Design review of the part built by this model. Coordinates are the model's own, in mm. Face numbers are marked on the shaded views. A direction names the side the tool comes from. Coordinates: 2 decimals unless noted, no trailing zeros. Order: outer loops, then holes, each group sorted by start corner. A loop starts at its lowest first (then second) coordinate and runs counter-clockwise, first axis right, second up. Notation, with made-up numbers: (64, 70.25) - (104, 70.25) arc R20 ccw to (104, 94.25) - close; hole circle Ø11 at (58.25, 65). An arc over 180 degrees is marked (long way). Write item = value, one per line. Start each with the question number.
```python
from build123d import *

# Parameters (mm, degrees)
SKETCH_1_W             = 14.3
SKETCH_1_H             = 17
EXTRUDE_1_DEPTH        = 6
SKETCH_3_W             = 0.2
SKETCH_3_H             = 0.2
EXTRUDE_3_DEPTH        = 1.2
PATTERN_LINEAR_1_COUNT = 19
PATTERN_LINEAR_1_PITCH = 0.5
SKETCH_4_W             = 0.3
SKETCH_4_H             = 0.5
EXTRUDE_4_DEPTH        = 6
CUT_EXTRUDE_1_DEPTH    = 10
SKETCH_8_W             = 0.883352336
SKETCH_8_H             = 11.931096145
EXTRUDE_6_DEPTH        = 5.2
CUT_EXTRUDE_4_DEPTH    = 24.382472068
EXTRUDE_7_DEPTH        = 2.1
EXTRUDE_7_DEPTH_BACK   = 5.2
SKETCH_12_W            = 1.5
SKETCH_12_H            = 0.486445161
SKETCH_12_W_2          = 1
SKETCH_13_R            = 0.6
EXTRUDE_8_DEPTH        = 2
SKETCH_15_R            = 1.25
EXTRUDE_9_DEPTH        = 0.4
SKETCH_16_W            = 4.2
SKETCH_16_H            = 9
EXTRUDE_10_DEPTH       = 3.3
FILLET_1_R             = 0.3


with BuildPart() as part:
    # 草图1 → 凸台-拉伸1 (new body)
    with BuildSketch(Plane.XY):
        with Locations((7.15, -8.5)):
            Rectangle(SKETCH_1_W, SKETCH_1_H)
    extrude(amount=EXTRUDE_1_DEPTH)

    # 草图3 → 凸台-拉伸3 (add)
    with BuildSketch(Plane(origin=(14.3, 0, 0), x_dir=(0, 0, -1), z_dir=(1, 0, 0))):
        with Locations((-0.1, -13.9)):
            Rectangle(SKETCH_3_W, SKETCH_3_H)
    extrude_3 = extrude(amount=EXTRUDE_3_DEPTH)

    # 阵列(线性)1: 凸台-拉伸3 ×19
    with Locations(*[(0, i * PATTERN_LINEAR_1_PITCH, 0) for i in range(1, PATTERN_LINEAR_1_COUNT)]):
        add(extrude_3)

    # 草图4 → 凸台-拉伸4 (add)
    with BuildSketch(Plane.XY.offset(6)):
        with Locations((0.15, 0.25)):
            Rectangle(SKETCH_4_W, SKETCH_4_H)
        with Locations((0.15, -17.25)):
            Rectangle(SKETCH_4_W, SKETCH_4_H)
    extrude(amount=-EXTRUDE_4_DEPTH)

    # 草图6 → 切除-拉伸1 (cut)
    with BuildSketch(Plane.ZY):
        Polygon((0.814275945, -1.576993803), (1.814275945, -0.576993803), (5.086945076, -0.576993803), (5.086945076, -16.573920601), (0.814275945, -16.573920601), align=None)
    extrude(amount=-CUT_EXTRUDE_1_DEPTH, mode=Mode.SUBTRACT)

    # 草图8 → 凸台-拉伸6 (add)
    with BuildSketch(Plane.ZY.offset(-10)):
        with Locations((2.941004683, -8.691870864)):
            Rectangle(SKETCH_8_W, SKETCH_8_H)
    extrude(amount=EXTRUDE_6_DEPTH)

    # 草图11 → 切除-拉伸4 (cut, through all)
    with BuildSketch(Plane(origin=(14.3, 0, 0), x_dir=(0, 0, -1), z_dir=(1, 0, 0))):
        Polygon((-2.744957318, 0.690687189), (0.440532754, -2.430132002), (0.440532754, 0.690687189), align=None)
    extrude(amount=-CUT_EXTRUDE_4_DEPTH, mode=Mode.SUBTRACT)

    # 草图12 → 凸台-拉伸7 (add, two sides: drawn at the far end of the back side and taken through both)
    with BuildSketch(Plane(origin=(0, 0, 0), x_dir=(-1, 0, 0), z_dir=(0, 0, -1)).offset(-EXTRUDE_7_DEPTH_BACK)):
        with Locations((-12.05, -16.75677742)):
            Rectangle(SKETCH_12_W, SKETCH_12_H)
        with Locations((-4.8, -16.75677742)):
            Rectangle(SKETCH_12_W_2, SKETCH_12_H)
        with Locations((-4.8, -0.243222581)):
            Rectangle(SKETCH_12_W_2, SKETCH_12_H)
        with Locations((-12.05, -0.243222581)):
            Rectangle(SKETCH_12_W, SKETCH_12_H)
    extrude(amount=EXTRUDE_7_DEPTH + EXTRUDE_7_DEPTH_BACK)

    # 草图13 → 凸台-拉伸8 (add)
    with BuildSketch(Plane(origin=(0, 0, 0), x_dir=(-1, 0, 0), z_dir=(0, 0, -1))):
        with Locations(Location((-4.5, -8.757432115, 0), (0, 0, 180))):
            Circle(SKETCH_13_R)
    extrude(amount=EXTRUDE_8_DEPTH)

    # 草图15 → 凸台-拉伸9 (add)
    with BuildSketch(Plane.ZY):
        with BuildLine():
            Line((6, -2.5), (13.5, -2.5))
            ThreePointArc((13.5, -2.5), (14.914213562, -3.085786438), (15.5, -4.5))
            Line((15.5, -4.5), (15.5, -12.5))
            ThreePointArc((15.5, -12.5), (14.914213562, -13.914213562), (13.5, -14.5))
            Line((13.5, -14.5), (6, -14.5))
            Line((6, -14.5), (6, -2.5))
        make_face()
        with Locations(Location((12.5, -8.5, 0), (0, 0, 270))):
            Circle(SKETCH_15_R, mode=Mode.SUBTRACT)
    extrude(amount=-EXTRUDE_9_DEPTH)

    # 草图16 → 凸台-拉伸10 (add)
    with BuildSketch(Plane.ZY):
        with Locations((3, -8.5)):
            Rectangle(SKETCH_16_W, SKETCH_16_H)
    extrude(amount=EXTRUDE_10_DEPTH)

    # 圆角1
    fillet_1_edges = [part.edges().sort_by_distance(p)[0] for p in [
        (0.3, 0.25, 6),
        (0.3, -17.25, 0),
        (0.3, -17.25, 6),
        (0.3, 0, 4.019978715),
        (0.4, -8.5, 6),
        (0.3, -17, 3),
        (2.3, -17, 0),
        (8.3, -17, 0),
        (13.55, -17, 0),
        (14.3, -17, 3),
        (7.3, -17, 6),
        (14.3, 0, 4.019978715),
        (14.3, -8.5, 6),
        (7.3, 0, 6),
    ]]
    fillet(fillet_1_edges, radius=FILLET_1_R - 0.0001)  # a hair under: the kernel refuses the full size


solid = part.part
```
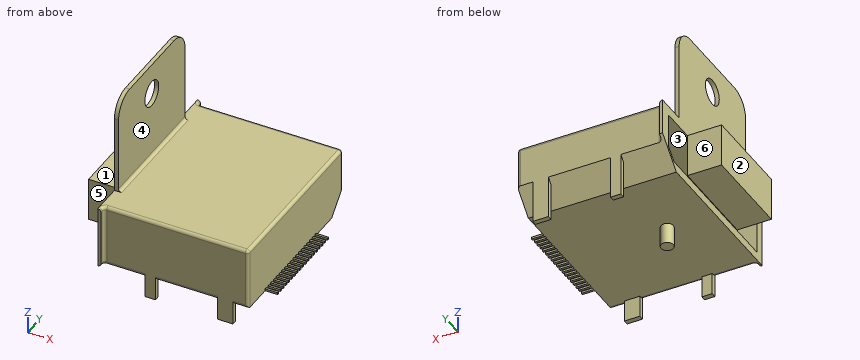
Item 1: For line 1 (Z direction, x = 0.2, y = -8.5); line 2 (Z direction, x = 1.25, y = -9); line 3 (Z direction, x = 8.5, y = -4.5), list the stretches that pass through material, from the lowest coordinate up.
Item 2: For P1, Ø3, axis at y = -13, z = 8, coming from the +X side; P2, Ø0.5, axis at y = -17, z = -1, coming from the +X side; P3, Ø4, axis at x = 13, z = 3.5, coming from the -Y side, all flat-tipped, find the tip position at first contact; note any pin that passes through.
Item 3: Add section D-D on z = -1. Give the boundary of the cut face in (x, y), plus the area to 3 significant figures.
Item 4: Add section C-C on z = 12.5. Give the boundary of the cut face in (x, y).
Item 5: For the marked faces 4, 5 and 6, list the 3-axis set-ups (+Z, -Z, +X, -X, +Y, -Y) from which the entire face can be reached by the end or side of a thin tool; tool diameter is ignored.
Item 6: Add section B-B on x = 2.5. Give the boundary of the cut face in (y, z), plus the area to 3 significant figures.
Item 7: Mouldability with a two-part tool opening along X and no side actions: class the marked faces 1, 2 and 3 as +X half, -X half, draft (parallel to the pull), parting line (faces both ways), or undercut.
Item 8: Add section A-A on x = 9. Give the boundary of the cut face in (y, z), plus the area to 3 significant figures.
Worked out:
q1.line_1 = 0 to 0.81, 5.09 to 11.25, 13.75 to 15.5
q1.line_2 = 0 to 0.81, 5.09 to 6
q1.line_3 = 0 to 0.81, 2.5 to 3.38, 5.09 to 6
q2.P1 = 0.4
q2.P2 = 12.8
q2.P3 = -17
q3.outline = circle Ø1.2 at (4.5, -8.76); (4.3, -17) - (5.3, -17) - (5.3, -16.51) - (4.3, -16.51) - close; (4.3, -0.49) - (5.3, -0.49) - (5.3, 0) - (4.3, 0) - close; (11.3, -17) - (12.8, -17) - (12.8, -16.51) - (11.3, -16.51) - close; (11.3, -0.49) - (12.8, -0.49) - (12.8, 0) - (11.3, 0) - close
q3.area = 3.56 mm2
q4.outline = (0, -14.5) - (0.4, -14.5) - (0.4, -9.75) - (0, -9.75) - close; (0, -7.25) - (0.4, -7.25) - (0.4, -2.5) - (0, -2.5) - close
q5.face_4 = +Z, +X, +Y, -Y
q5.face_5 = +Z, -Z, -X, -Y
q5.face_6 = +Z, -Z, -X, +Y
q6.outline = (-17, 0.3) arc R0.3 ccw to (-16.7, 0) - (-2, 0) - (0, 2.04) - (0, 5.7) arc R0.3 ccw to (-0.3, 6) - (-16.7, 6) arc R0.3 ccw to (-17, 5.7) - close; hole (-16.57, 0.81) - (-1.58, 0.81) - (-0.58, 1.81) - (-0.58, 5.09) - (-16.57, 5.09) - close
q6.area = 32.1 mm2
q7.face_1 = draft
q7.face_2 = -X half
q7.face_3 = undercut
q8.outline = (-17, 0.3) arc R0.3 ccw to (-16.7, 0) - (-2, 0) - (0, 2.04) - (0, 5.7) arc R0.3 ccw to (-0.3, 6) - (-16.7, 6) arc R0.3 ccw to (-17, 5.7) - close; (-14.66, 2.5) - (-2.73, 2.5) - (-2.73, 3.38) - (-14.66, 3.38) - close; hole (-16.57, 0.81) - (-1.58, 0.81) - (-0.58, 1.81) - (-0.58, 5.09) - (-16.57, 5.09) - close
q8.area = 42.6 mm2
